CAD build for the part. Positions are in the model's coordinates, mm. Face numbers are marked on the shaded views. A direction names the side the tool comes from. Coordinates: 2 decimals unless noted, no trailing zeros. Loops run counter-clockwise (first coordinate to the right, second up) from the corner with the lowest first, then second, coordinate; pieces in that order, holes last. Notation, with made-up numbers: (-29, 22) - (-8, 22) arc R26 ccw to (-8, 52) - close; hole circle Ø6 at (63.25, 56). An arc over 180 degrees is marked (long way). Put each result on its own line as item: value.
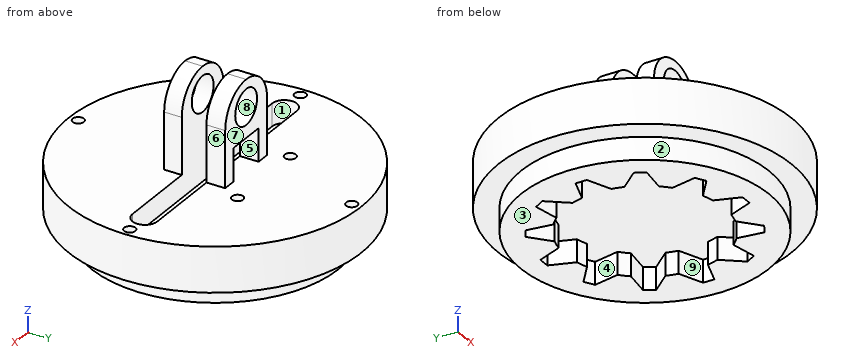
```python
from build123d import *

# Parameters (mm, degrees)
SKETCH2_R           = 65
BOSS_EXTRUDE1_DEPTH = 20
SKETCH4_R           = 55
BOSS_EXTRUDE2_DEPTH = 10
SHELL1_T            = -20
CUT_EXTRUDE4_DEPTH  = 10
CIRPATTERN3_COUNT   = 12
CUT_EXTRUDE5_DEPTH  = 10
SKETCH13_R          = 2.5
CUT_EXTRUDE7_DEPTH  = 10
CIRPATTERN4_COUNT   = 4
SKETCH14_W          = 30
SKETCH14_H          = 8.321649063
SKETCH14_H_2        = 7.815978975
BOSS_EXTRUDE3_DEPTH = 40
SKETCH15_R          = 7.825
CUT_EXTRUDE8_DEPTH  = 60
FILLET3_R           = 15
SKETCH16_W          = 17.850622268
SKETCH16_H          = 14.602901006
CUT_EXTRUDE9_DEPTH  = 10
SKETCH19_R          = 2.5
CUT_EXTRUDE10_DEPTH = 10


with BuildPart() as part:
    # Sketch2 → Boss-Extrude1 (new body)
    with BuildSketch(Plane(origin=(0, 0, 0), x_dir=(0, 1, 0), z_dir=(0, 0, 1))):
        with Locations(Location((0, 0, 0), (0, 0, 270))):
            Circle(SKETCH2_R)
    extrude(amount=BOSS_EXTRUDE1_DEPTH)

    # Sketch4 → Boss-Extrude2 (add)
    with BuildSketch(Plane(origin=(0, 0, 0), x_dir=(1, 0, 0), z_dir=(0, 0, -1))):
        with Locations(Location((0, 0, 0), (0, 0, 180))):
            Circle(SKETCH4_R)
    extrude(amount=BOSS_EXTRUDE2_DEPTH)

    # Shell1
    shell1_openings = [part.faces().sort_by_distance(p)[0] for p in [
        (0, 0, -10),
    ]]
    offset(amount=SHELL1_T, openings=shell1_openings, kind=Kind.INTERSECTION)

    # Sketch11 → Cut-Extrude4 (cut)
    with BuildSketch(Plane(origin=(0, 0, -10), x_dir=(1, 0, 0), z_dir=(0, 0, -1))):
        Polygon((-0.14294056, 45.151393391), (2.152952162, 45.151393391), (6.37913534, 34.41375644), (-6.666711392, 34.359204869), (-2.847047838, 45.151393391), align=None)
    cut_extrude4 = extrude(amount=-CUT_EXTRUDE4_DEPTH, mode=Mode.SUBTRACT)

    # CirPattern3: Cut-Extrude4 ×12 about axis
    cirpattern3_axis = Axis((0, 0, 0), (0, 0, 1))
    for i in range(1, CIRPATTERN3_COUNT):
        add(cut_extrude4.rotate(cirpattern3_axis, i * 360 / CIRPATTERN3_COUNT), mode=Mode.SUBTRACT)

    # Sketch12 → Cut-Extrude5 (cut)
    with BuildSketch(Plane.XY.offset(20)):
        with BuildLine():
            Line((-49.724225287, 5.5), (50.275774713, 5.5))
            ThreePointArc((50.275774713, 5.5), (55.775774713, 0), (50.275774713, -5.5))
            Line((50.275774713, -5.5), (-49.724225287, -5.5))
            ThreePointArc((-49.724225287, -5.5), (-55.224225287, 0), (-49.724225287, 5.5))
        make_face()
    extrude(amount=-CUT_EXTRUDE5_DEPTH, mode=Mode.SUBTRACT)

    # Sketch13 → Cut-Extrude7 (cut)
    with BuildSketch(Plane.XY.offset(20)):
        with Locations((0.158711009, 60.870900594)):
            Circle(SKETCH13_R)
    cut_extrude7 = extrude(amount=-CUT_EXTRUDE7_DEPTH, mode=Mode.SUBTRACT)

    # CirPattern4: Cut-Extrude7 ×4 about axis
    cirpattern4_axis = Axis((0, 0, 0), (0, 0, 1))
    for i in range(1, CIRPATTERN4_COUNT):
        add(cut_extrude7.rotate(cirpattern4_axis, i * 360 / CIRPATTERN4_COUNT), mode=Mode.SUBTRACT)

    # Sketch14 → Boss-Extrude3 (add)
    with BuildSketch(Plane.XY.offset(20)):
        with Locations((0, 9.660824532)):
            Rectangle(SKETCH14_W, SKETCH14_H)
        with Locations((0, -9.407989488)):
            Rectangle(SKETCH14_W, SKETCH14_H_2)
    extrude(amount=BOSS_EXTRUDE3_DEPTH)

    # Sketch15 → Cut-Extrude8 (cut)
    with BuildSketch(Plane.XZ.offset(13.315978975)):
        with Locations(Location((0, 48.024835591, 0), (0, 0, 270))):
            Circle(SKETCH15_R)
    extrude(amount=-CUT_EXTRUDE8_DEPTH, mode=Mode.SUBTRACT)

    # Fillet3
    fillet3_edges = [part.edges().sort_by_distance(p)[0] for p in [
        (-15, -9.407989488, 60),
        (-15, 9.660824531, 60),
        (15, 9.660824531, 60),
        (15, -9.407989488, 60),
    ]]
    fillet(fillet3_edges, radius=FILLET3_R - 0.0001)  # a hair under: the kernel refuses the full size

    # Sketch16 → Cut-Extrude9 (cut)
    with BuildSketch(Plane(origin=(0, 13.821649063, 0), x_dir=(-1, 0, 0), z_dir=(0, 1, 0))):
        with Locations((0.019760197, 27.301450503)):
            Rectangle(SKETCH16_W, SKETCH16_H)
    extrude(amount=-CUT_EXTRUDE9_DEPTH, mode=Mode.SUBTRACT)

    # Sketch19 → Cut-Extrude10 (cut)
    with BuildSketch(Plane.XY.offset(20)):
        with Locations((-18.87834994, 21.74381377)):
            Circle(SKETCH19_R)
        with Locations((18.87834994, 21.74381377)):
            Circle(SKETCH19_R)
    extrude(amount=-CUT_EXTRUDE10_DEPTH, mode=Mode.SUBTRACT)


solid = part.part
```
Q1. Tool access for the marked faces 5, 6, 7, 8 and 9: list every direction of +Z, -Z, +X, -X, +Y, -Y with a clear straight run to the whole face (end or side of a thin tool).
Determined:
face 5: +Y
face 6: +Z, +X, +Y, -Y
face 7: +Z, +X, -X, +Y
face 8: +Y, -Y
face 9: -Z
Q2. Slice it at C-C, the plane x = 18.5. Give the cut face in (y, z), then the cut area to 3 significant figures.
Determined:
outline: (-62.31, 0) - (-51.8, 0) - (-51.8, -10) - (-39.15, -10) - (-39.15, 0) - (38.42, 0) - (38.42, -10) - (51.8, -10) - (51.8, 0) - (62.31, 0) - (62.31, 20) - (24.22, 20) - (24.22, 10) - (19.27, 10) - (19.27, 20) - (5.5, 20) - (5.5, 10) - (-5.5, 10) - (-5.5, 20) - (-62.31, 20) - close
area: 2,590 mm2
Q3. Slice it at B-B, the plane y = 0. Give the cut face in (x, z), then the cut area to 3 significant figures.
Determined:
outline: (-65, 0) - (-55, 0) - (-55, -10) - (-45.15, -10) - (-45.15, 0) - (45.15, 0) - (45.15, -10) - (55, -10) - (55, 0) - (65, 0) - (65, 20) - (63.37, 20) - (63.37, 10) - (58.38, 10) - (58.38, 20) - (55.78, 20) - (55.78, 10) - (-55.22, 10) - (-55.22, 20) - (-58.38, 20) - (-58.38, 10) - (-63.37, 10) - (-63.37, 20) - (-65, 20) - close
area: 1,590 mm2
Q4. Wall check: L1, parallel to Y at x = -7, z = 39; L2, parallel to Z at x = 23, y = -32; L3, parallel to Z at x = 53, y = 8.5. Give the ranges that are in metal, low to high. Write a range as from..to.
Determined:
L1: -13.32..-5.5, 5.5..13.82
L2: 0..20
L3: -10..20
Q5. Mould opens along X. For the marked faces 1, 2, 3 and 4 say: +X half, -X half, draft (parallel to the pull), parting line (faces both ways), or undercut.
Determined:
face 1: undercut
face 2: parting line
face 3: draft
face 4: undercut
Q6. Slice it at A-A, the plane z = 18. Give the cut face in (x, y), then the cut area to 3 significant figures.
Determined:
outline: circle Ø130 at (0, 0); hole circle Ø5 at (-60.87, 0.16); hole (-49.72, -5.5) - (50.28, -5.5) arc R5.5 ccw to (50.28, 5.5) - (-49.72, 5.5) arc R5.5 ccw to start; hole circle Ø5 at (-18.88, 21.74); hole circle Ø5 at (-0.16, -60.87); hole circle Ø5 at (0.16, 60.87); hole circle Ø5 at (18.88, 21.74); hole circle Ø5 at (60.87, -0.16)
area: 12,000 mm2
Q7. Pin check, flat tips, straight feed: pin 1 Ø4.5 at (x, y) = (-18.88, 21.74) entering from +Z; pin 2 Ø12 at (y, z) = (-18, 25.5) entering from +X; pin 3 Ø5 at (x, y) = (-42, 14.5) entering from +Z. Stop position of each tip, or through.
Determined:
pin 1: z = 10
pin 2: x = 63.1
pin 3: z = 20
